Autodesk Inventor part; units mm, degrees
ref_plane "YZ Plane" through (0, 0, 0) normal (1, 0, 0) x (0, 1, 0)
ref_plane "XZ Plane" through (0, 0, 0) normal (0, 1, 0) x (-1, 0, 0)
ref_plane "XY Plane" through (0, 0, 0) normal (0, 0, 1) x (1, 0, 0)
sketch "Sketch1" plane through (0, 0, 0) normal (0, 0, 1) x (1, 0, 0)
  circle A0 centre (0, 0) radius 3.5
  dimension "d0" = 7
extrude "Extrusion1" add sketch "Sketch1" along normal blind 50
sketch "Sketch2" plane through (0, 0, 50) normal (0, 0, 1) x (1, 0, 0)
  circle A0 centre (0, 0) radius 3.5
  circle A1 centre (0, 0) radius 2.495
  dimension "d3" = 4.99
extrude "Extrusion2" add sketch "Sketch2" along normal blind 2 contours A1
sketch "Sketch3" plane through (0, 0, 0) normal (0, 0, -1) x (-1, 0, 0)
  circle A0 centre (0, 0) radius 3.5
  circle A1 centre (0, 0) radius 2.495
extrude "Extrusion3" add sketch "Sketch3" along normal blind 2 contours A1
properties part number "Steunpaal"
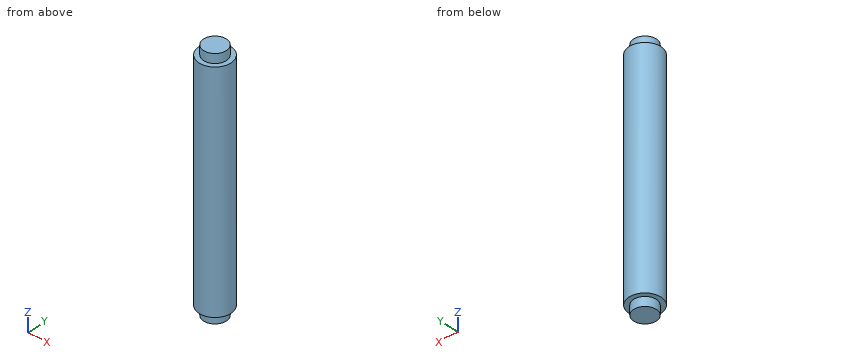
The listing builds one solid part. Answer for the finished solid, in the listing's coordinates (mm). Round coordinates to 2 decimals unless told otherwise and drop trailing zeros. Write each loop counter-clockwise with the first axis right and the second up, starting at its lowest first coordinate (ties: lowest second). Pieces come first, ordered by that corner, then holes. Notation, with made-up numbers: (-36, 48.5) -> (-4, 48.5) arc R13 ccw to (-4, 59.5) -> close; hole circle Ø5 at (-8.75, 85.25). An arc over 180 degrees is marked (long way). Answer as a JSON object with one key per item and string values. Group by question number.
Q1. Section A-A (x = 0) is taken. Write down the section's boundary in (y, z) (3 decimals), plus the area to 3 significant figures.
Q2. Section C-C (z = 42) is taken. Write down the section's boundary in (x, y), plus the area to 3 significant figures.
Q3. Straight lines are drawn through the part: line 1 along Z through (x, y) = (1.75, -2.25); line 2 along X through (y, z) = (0.25, 10); line 3 along Y through (x, z) = (2.5, 28.5). For each, find the intervals that lie inside material, in ascending order.
Q4. Each of these flat-tipped pins is pushed along its axis until it touches: pin 1 Ø1.5 at (x, z) = (-2.5, 14.5) entering from -Y; pin 2 Ø1 at (x, z) = (2.5, 27.5) entering from -Y. Where does it stop, or does it pass through?
Check values:
{
 "1": {"outline": "(-3.5, 0) -> (-2.495, 0) -> (-2.495, -2) -> (2.495, -2) -> (2.495, 0) -> (3.5, 0) -> (3.5, 50) -> (2.495, 50) -> (2.495, 52) -> (-2.495, 52) -> (-2.495, 50) -> (-3.5, 50) -> close", "area": "370 mm^2"},
 "2": {"outline": "circle Ø7 at (0, 0)", "area": "38.5 mm^2"},
 "3": {"line 1": "0 to 50", "line 2": "-3.49 to 3.49", "line 3": "-2.45 to 2.45"},
 "4": {"pin 1": "y = -3.03", "pin 2": "y = -2.87"}
}
